Source: CAD feature listing. Evaluate the final solid. Frame: model axes, mm. A direction names the side the tool comes from. Give positions to 0.01 mm unless a question says otherwise; leave off trailing zeros. Write each loop counter-clockwise with the first axis right and the second up, starting at its lowest first coordinate (ties: lowest second). Pieces come first, ordered by that corner, then holes. Notation, with made-up numbers: M 10.25,-36.75 L 37.25,-36.75 A23 ccw 37.25,-24.75 Z; hole C 40.5,17 d4. An arc over 180 degrees is marked long. Answer as a JSON object with one key per item and string values. Group by question number.
```python
from build123d import *

# Parameters (mm, degrees)
F1_DEPTH = 16
F2_R     = 3
F3_DEPTH = 16.001
F4_R     = 3
F5_DEPTH = 6


with BuildPart() as f1:
    # F0 (on Top) → F1 (new body)
    with BuildSketch(Plane.XY):
        with BuildLine():
            ThreePointArc((9.3561974046, -1.7852717232), (9.4827054494, -0.8966171761), (9.525, 0))
            ThreePointArc((9.525, 0), (9.4827054494, 0.8966171761), (9.3561974046, 1.7852717232))
            ThreePointArc((9.3561974046, 1.7852717232), (7.9216471704, 2.5738991923), (8.6186790933, 4.0551196883))
            ThreePointArc((8.6186790933, 4.0551196883), (7.7058868714, 5.5986545281), (6.5199663128, 6.9437500156))
            ThreePointArc((6.5199663128, 6.9437500156), (4.8958471982, 6.738555569), (4.5891183065, 8.3465932074))
            ThreePointArc((4.5891183065, 8.3465932074), (2.9433868714, 9.0588133177), (1.193329695, 9.4499518115))
            ThreePointArc((1.193329695, 9.4499518115), (0, 8.3293127534), (-1.193329695, 9.4499518115))
            ThreePointArc((-1.193329695, 9.4499518115), (-2.9433868714, 9.0588133177), (-4.5891183065, 8.3465932074))
            ThreePointArc((-4.5891183065, 8.3465932074), (-4.4504477573, 8.039487236), (-4.4029672815, 7.7058868714))
            ThreePointArc((-4.4029672815, 7.7058868714), (-5.1936438859, 6.5808827064), (-6.5199663128, 6.9437500156))
            ThreePointArc((-6.5199663128, 6.9437500156), (-7.7058868714, 5.5986545281), (-8.6186790933, 4.0551196883))
            ThreePointArc((-8.6186790933, 4.0551196883), (-8.0698919683, 3.6154750772), (-7.8631260711, 2.9433868714))
            ThreePointArc((-7.8631260711, 2.9433868714), (-8.3259799016, 1.9985995007), (-9.3561974046, 1.7852717232))
            ThreePointArc((-9.3561974046, 1.7852717232), (-9.525, 0), (-9.3561974046, -1.7852717232))
            ThreePointArc((-9.3561974046, -1.7852717232), (-8.3259799016, -1.9985995007), (-7.8631260711, -2.9433868714))
            ThreePointArc((-7.8631260711, -2.9433868714), (-8.0698919683, -3.6154750772), (-8.6186790933, -4.0551196883))
            ThreePointArc((-8.6186790933, -4.0551196883), (-7.7058868714, -5.5986545281), (-6.5199663128, -6.9437500156))
            ThreePointArc((-6.5199663128, -6.9437500156), (-5.1936438859, -6.5808827064), (-4.4029672815, -7.7058868714))
            ThreePointArc((-4.4029672815, -7.7058868714), (-4.4504477573, -8.039487236), (-4.5891183065, -8.3465932074))
            ThreePointArc((-4.5891183065, -8.3465932074), (-2.9433868714, -9.0588133177), (-1.193329695, -9.4499518115))
            ThreePointArc((-1.193329695, -9.4499518115), (0, -8.3293127534), (1.193329695, -9.4499518115))
            ThreePointArc((1.193329695, -9.4499518115), (2.9433868714, -9.0588133177), (4.5891183065, -8.3465932074))
            ThreePointArc((4.5891183065, -8.3465932074), (4.8958471982, -6.738555569), (6.5199663128, -6.9437500156))
            ThreePointArc((6.5199663128, -6.9437500156), (7.7058868714, -5.5986545281), (8.6186790933, -4.0551196883))
            ThreePointArc((8.6186790933, -4.0551196883), (7.9216471704, -2.5738991923), (9.3561974046, -1.7852717232))
        make_face()
    extrude(amount=F1_DEPTH)

    # F2 (on face) → F3 (cut, through all)
    with BuildSketch(Plane.XY.offset(16)):
        Circle(F2_R)
    extrude(amount=-F3_DEPTH, mode=Mode.SUBTRACT)

    # F4 (on face) → F5 (cut)
    with BuildSketch(Plane.XY.offset(16)):
        Polygon((2.8867513459, -5), (5.7735026919, 0), (2.8867513459, 5), (-2.8867513459, 5), (-5.7735026919, 0), (-2.8867513459, -5), align=None)
        Circle(F4_R, mode=Mode.SUBTRACT)
    extrude(amount=-F5_DEPTH, mode=Mode.SUBTRACT)


solid = f1.part
```
(1) Section A-A, the plane x = 0. Return loops of the section in (y, z).
(2) Contact query for flat-ended pins moving along their axis: pin 1 Ø4 at (x, z) = (4.5, 11) entering from -Y; pin 2 Ø5 at (x, z) = (-6, 8.5) entering from -Y; pin 3 Ø5 at (x, z) = (-4, 4.5) entering from -Y. Output: stop coordinate, or through.
(3) Section D-D, the plane z = 3.25. Return loops of the section in (x, y) (3 decimals), plus the area to 3 significant figures.
(4) Ray query, L1, parallel to Y at x = 0, z = 6.75; L2, parallel to Z at x = 5, y = 0; L3, parallel to Y at x = 8.25, z = 14. Return the intervals inside material, ascending. Write a range as [from, to].
(5) Section C-C, the plane y = -2.5. Return loops of the section in (x, z), plus the area to 3 significant figures.
(6) Pull-direction query (Y, two-part tool) for faces 3 (the flat face through (-4.31, 2.535, 13.042)), 4 (the cylindrical face through (-7.69, 5.62, 7.89)), 5 (the flat face through (2.5, 2.3, 10)), 6 (the cylindrical face through (-0.03, -8.33, 7.89)); classes: pulls with the +Y half, pulls with the -Y half, needs draft (parallel to the pull), parting line crosses it, or undercut.
(7) Access query for faces 1 (the cylindrical face through (4.88, -6.75, 7.89)), 2 (the flat face through (0, -5, 13)). Directions: +Z, -Z, +X, -X, +Y, -Y. A direction counts if a zero-diameter tool reaches every point of the face in a straight line with its end or side. Return the directions, or none.
Reported:
{
 "1": {"outline": "M -8.33,0 L -3,0 L -3,10 L -5,10 L -5,16 L -8.33,16 Z; M 3,0 L 8.33,0 L 8.33,16 L 5,16 L 5,10 L 3,10 Z"},
 "2": {"pin 1": "stops at y = -9.19", "pin 2": "stops at y = -8.86", "pin 3": "stops at y = -9.41"},
 "3": {"outline": "M -9.356,-1.785 A1.196 cw -8.619,-4.055 A9.525 ccw -6.52,-6.944 A1.196 cw -4.589,-8.347 A9.525 ccw -1.193,-9.45 A1.196 cw 1.193,-9.45 A9.525 ccw 4.589,-8.347 A1.196 cw 6.52,-6.944 A9.525 ccw 8.619,-4.055 A1.196 cw 9.356,-1.785 A9.525 ccw 9.356,1.785 A1.196 cw 8.619,4.055 A9.525 ccw 6.52,6.944 A1.196 cw 4.589,8.347 A9.525 ccw 1.193,9.45 A1.196 cw -1.193,9.45 A9.525 ccw -4.589,8.347 A1.196 cw -6.52,6.944 A9.525 ccw -8.619,4.055 A1.196 cw -9.356,1.785 A9.525 ccw Z; hole C 0,0 d6", "area": "235 mm2"},
 "4": {"L1": "y = [-8.33, -3], [3, 8.33]", "L2": "z = [0, 10]", "L3": "y = [-4.76, -3.82], [-2.06, 2.06], [3.82, 4.76]"},
 "5": {"outline": "M -7.95,0 L -1.66,0 L -1.66,10 L -4.33,10 L -4.33,16 L -7.95,16 Z; M 1.66,0 L 7.95,0 L 7.95,16 L 4.33,16 L 4.33,10 L 1.66,10 Z", "area": "169 mm2"},
 "6": {"face 3": "undercut", "face 4": "pulls with the +Y half", "face 5": "undercut", "face 6": "pulls with the -Y half"},
 "7": {"face 1": "+Z, -Z", "face 2": "+Z"}
}
